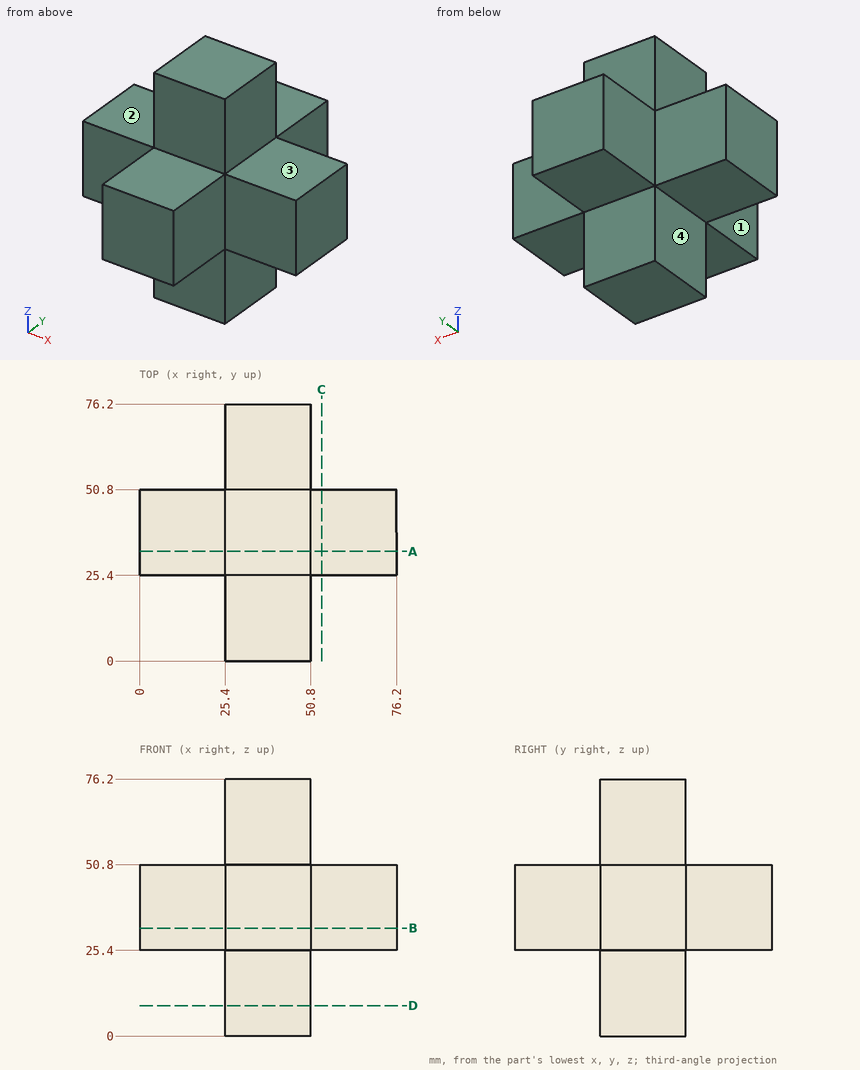
Answer from the drawing. Dimensions are ordinates in mm from the lowest x, y and z of the part. A direction names the side the tool comes from. Give positions to 0.01 mm unless a question says otherwise; leave off trailing zeros. Write each loop counter-clockwise with the first axis right and the second up, starting at its lowest first coordinate (ties: lowest second). Pieces come first, ordered by that corner, then holes. Notation, with made-up numbers: M 26,55 L 50,55 A21 ccw 50,77 Z; hole C -38,21 d11. An arc over 180 degrees is marked long. Answer as CSV lines item,"result".
Q1. A cutting plane is placed at C-C on x = 54. Write down the section's boundary in (y, z), plus the area to 3 significant figures.
A:
outline,"M 25.4,25.4 L 50.8,25.4 L 50.8,50.8 L 25.4,50.8 Z"
area,"645 mm²"
Q2. A tool of negligible diameter and unlimited length cuts with its end or side. For the marked faces 1, 2, 3 and 4, from which of +Z, -Z, +X, -X, +Y, -Y can it reach the whole face along a straight path? Write none if from no direction.
A:
face 1,"+Z, -Z, -X, -Y"
face 2,"+Z, -X, +Y, -Y"
face 3,"+Z, +X, +Y, -Y"
face 4,"-Z, -X, +Y, -Y"
Q3. A cutting plane is placed at A-A on y = 32.5. Write down the section's boundary in (x, z), plus the area to 3 significant figures.
A:
outline,"M 0,25.4 L 25.4,25.4 L 25.4,0 L 50.8,0 L 50.8,25.4 L 76.2,25.4 L 76.2,50.8 L 50.8,50.8 L 50.8,76.2 L 25.4,76.2 L 25.4,50.8 L 0,50.8 Z"
area,"3,230 mm²"
Q4. Given P1, Ø7.5, axis at x = 34, y = 18.5, coming from the -Z side; P2, Ø10, axis at y = 51.5, z = 64.5, coming from the -X side; P3, Ø7.5, axis at x = 7.5, y = 35.5, coming from the +Z side, each flat-ended and moving along its own axis, determine where each tip first touches the part or whether it passes through.
A:
P1,"stops at z = 25.4"
P2,"stops at x = 25.4"
P3,"stops at z = 50.8"
Q5. Find the intervals of material crossed by probe 1 along Z at (x, y) = (34, 24.5), in increasing order. Write a range as [from, to].
A:
probe 1,"z = [25.4, 50.8]"
